Geometry: final body of the model. Coordinates: model frame, mm. Face numbers are marked on the shaded views. A direction names the side the tool comes from. Give positions to 0.01 mm unless a question says otherwise; leave off trailing zeros. Write each loop counter-clockwise with the first axis right and the second up, starting at its lowest first coordinate (ties: lowest second). Pieces come first, ordered by that corner, then holes.
from build123d import *

# Parameters (mm, degrees)
BOSS_EXTRUDE1_DEPTH = 31
SKETCH2_W           = 27
SKETCH2_H           = 3
CUT_EXTRUDE1_DEPTH  = 47.54655438
SKETCH3_W           = 25
SKETCH3_H           = 42.4
CUT_EXTRUDE2_DEPTH  = 46.707660351
FILLET1_R           = 10


with BuildPart() as part:
    # Sketch1 → Boss-Extrude1 (new body)
    with BuildSketch(Plane(origin=(0, 0, 0), x_dir=(0, 0, -1), z_dir=(1, 0, 0))):
        with BuildLine():
            Line((-24.2, 0), (24.2, 0))
            Line((24.2, 0), (24.2, 0.8))
            Line((24.2, 0.8), (26.2, 0.8))
            Line((26.2, 0.8), (26.2, -1.574624922))
            Line((26.2, -1.574624922), (33.093654271, -2.790162166))
            Line((33.093654271, -2.790162166), (32.572709738, -5.744585425))
            Line((32.572709738, -5.744585425), (22.5, -3.968494929))
            ThreePointArc((22.5, -3.968494929), (0, -2), (-22.5, -3.968494929))
            Line((-22.5, -3.968494929), (-32.572709738, -5.744585425))
            Line((-32.572709738, -5.744585425), (-33.093654271, -2.790162166))
            Line((-33.093654271, -2.790162166), (-26.2, -1.574624922))
            Line((-26.2, -1.574624922), (-26.2, 0.8))
            Line((-26.2, 0.8), (-24.2, 0.8))
            Line((-24.2, 0.8), (-24.2, 0))
        make_face()
    extrude(amount=BOSS_EXTRUDE1_DEPTH)

    # Sketch2 → Cut-Extrude1 (cut, through all)
    with BuildSketch(Plane(origin=(0, 2.953319706, -0.520749947), x_dir=(1, 0, 0), z_dir=(0, 0.9848077530122087, -0.17364817766692767))):
        with Locations((15.5, 29.575393877)):
            Rectangle(SKETCH2_W, SKETCH2_H)
    cut_extrude1 = extrude(amount=-CUT_EXTRUDE1_DEPTH, mode=Mode.SUBTRACT)

    # Mirror1: Cut-Extrude1 across plane
    add(cut_extrude1.mirror(Plane.XY), mode=Mode.SUBTRACT)

    # Sketch3 → Cut-Extrude2 (cut, through all)
    with BuildSketch(Plane(origin=(0, 0, 0), x_dir=(1, 0, 0), z_dir=(0, 1, 0))):
        with Locations((15.5, 0)):
            Rectangle(SKETCH3_W, SKETCH3_H)
    extrude(amount=-CUT_EXTRUDE2_DEPTH, mode=Mode.SUBTRACT)

    # Fillet1
    fillet1_edges = [part.edges().sort_by_distance(p)[0] for p in [
        (28, -1.873042869, -21.2),
        (28, -1.873042869, 21.2),
    ]]
    fillet(fillet1_edges, radius=FILLET1_R)


solid = part.part
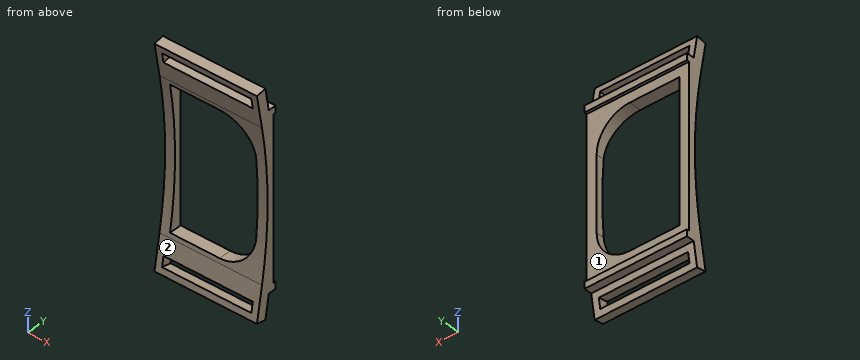
Q1. Section C-C on z = -14.5. Output: boundary loops of the cut face in (x, y), plus the area to 3 significant figures.
Filled sheet:
outline: (0, -2.81) - (3, -2.81) - (3, 0) - (0, 0) - close; (27.44, -2.81) - (31, -2.81) - (31, 0) - (27.44, 0) - close
area: 18.5 mm2
Q2. Section B-B on z = -7. Output: boundary loops of the cut face in (x, y), plus the area to 3 significant figures.
Filled sheet:
outline: (0, -2.19) - (3, -2.19) - (3, 0) - (0, 0) - close; (28, -2.19) - (31, -2.19) - (31, 0) - (28, 0) - close
area: 13.1 mm2
Q3. Ray query, line 1 along Z through (x, y) = (5, 0.25); line 2 along X through (y, z) = (-1.75, 2.5); line 3 along Z through (x, y) = (11.5, -0.5). Return the intervals inside material, ascending.
Filled sheet:
line 1: z = -26.2 to -24.2, 24.2 to 26.2
line 2: x = 0 to 3, 28 to 31
line 3: z = -26.2 to -21.2, 21.2 to 26.2
Q4. Section D-D on x = 23. Output: boundary loops of the cut face in (y, z), plus the area to 3 significant figures.
Filled sheet:
outline: (-5.74, -32.57) - (-2.79, -33.09) - (-2.44, -31.12) - (-5.4, -30.6) - close; (-5.74, 32.57) - (-5.4, 30.6) - (-2.44, 31.12) - (-2.79, 33.09) - close; (-4.88, -27.65) - (-1.92, -28.17) - (-1.57, -26.2) - (0.8, -26.2) - (0.8, -24.2) - (0, -24.2) - (0, -19.86) - (-3.53, -19.86) arc R129.57 cw to (-3.97, -22.5) - close; (-4.88, 27.65) - (-3.97, 22.5) arc R129.57 cw to (-3.53, 19.86) - (0, 19.86) - (0, 24.2) - (0.8, 24.2) - (0.8, 26.2) - (-1.57, 26.2) - (-1.92, 28.17) - close
area: 77.2 mm2
Q5. Pin query (flat end, axial travel): P1, Ø3, axis at x = 13, z = -24.5, coming from the -Y side; P2, Ø1, axis at x = 23, y = -3.5, coming from the -Z side; P3, Ø1.2, axis at x = 20.5, y = 0, coming from the +Z side. Return the tip coordinate at first contact, or that it passes through.
Filled sheet:
P1: stops at y = -4.59
P2: stops at z = -33.06
P3: stops at z = 26.2
Q6. Section A-A on x = 13.5. Output: boundary loops of the cut face in (y, z).
Filled sheet:
outline: (-5.74, -32.57) - (-2.79, -33.09) - (-2.44, -31.12) - (-5.4, -30.6) - close; (-5.74, 32.57) - (-5.4, 30.6) - (-2.44, 31.12) - (-2.79, 33.09) - close; (-4.88, -27.65) - (-1.92, -28.17) - (-1.57, -26.2) - (0.8, -26.2) - (0.8, -24.2) - (0, -24.2) - (0, -21.2) - (-3.75, -21.2) arc R129.57 cw to (-3.97, -22.5) - close; (-4.88, 27.65) - (-3.97, 22.5) arc R129.57 cw to (-3.75, 21.2) - (0, 21.2) - (0, 24.2) - (0.8, 24.2) - (0.8, 26.2) - (-1.57, 26.2) - (-1.92, 28.17) - close
Q7. Access query for the marked faces 1 and 2. Directions: +Z, -Z, +X, -X, +Y, -Y. A direction counts if a zero-diameter tool reaches every point of the face in a straight line with its end or side. Return the directions, or none.
Filled sheet:
face 1: +X, -X, +Y
face 2: +X, -X, -Y
